from build123d import *

# Parameters (mm, degrees)
SKETCH2_R               = 95
SKETCH2_R_2             = 75
BOSS_EXTRUDE1_DEPTH     = 5
SKETCH3_R               = 87
SKETCH3_R_2             = 84
BOSS_EXTRUDE2_DEPTH     = 10
SKETCH4_R               = 78
SKETCH4_R_2             = 75
BOSS_EXTRUDE3_DEPTH     = 70
CUT_EXTRUDE3_DEPTH      = 161.23420359
CUT_EXTRUDE3_DEPTH_BACK = 161.23420359
SKETCH6_W               = 10
SKETCH6_H               = 12
CUT_EXTRUDE4_DEPTH      = 161.23420359
CUT_EXTRUDE4_DEPTH_BACK = 161.23420359
SKETCH7_W               = 10
SKETCH7_H               = 12


with BuildPart() as part:
    # Sketch2 → Boss-Extrude1 (new body)
    with BuildSketch(Plane.XY):
        Circle(SKETCH2_R)
        Circle(SKETCH2_R_2, mode=Mode.SUBTRACT)
    extrude(amount=BOSS_EXTRUDE1_DEPTH)

    # Sketch3 → Boss-Extrude2 (add)
    with BuildSketch(Plane.XY):
        Circle(SKETCH3_R)
        Circle(SKETCH3_R_2, mode=Mode.SUBTRACT)
    extrude(amount=BOSS_EXTRUDE2_DEPTH)

    # Sketch4 → Boss-Extrude3 (add)
    with BuildSketch(Plane.XY.offset(5)):
        Circle(SKETCH4_R)
        Circle(SKETCH4_R_2, mode=Mode.SUBTRACT)
    extrude(amount=BOSS_EXTRUDE3_DEPTH)

    # Sketch6 → Cut-Extrude3 (cut, two sides: drawn at the far end of the back side and taken through both)
    with BuildSketch(Plane(origin=(10, 0, 0), x_dir=(0, 0, -1), z_dir=(1, 0, 0)).offset(-CUT_EXTRUDE3_DEPTH_BACK)):
        with Locations((-40, 40)):
            Rectangle(SKETCH6_W, SKETCH6_H)
    extrude(amount=CUT_EXTRUDE3_DEPTH + CUT_EXTRUDE3_DEPTH_BACK, mode=Mode.SUBTRACT)

    # Sketch7 → Cut-Extrude4 (cut, two sides: drawn at the far end of the back side and taken through both)
    with BuildSketch(Plane(origin=(10, 0, 0), x_dir=(0, 0, -1), z_dir=(1, 0, 0)).offset(-CUT_EXTRUDE4_DEPTH_BACK)):
        with Locations((-40, -40)):
            Rectangle(SKETCH7_W, SKETCH7_H)
    extrude(amount=CUT_EXTRUDE4_DEPTH + CUT_EXTRUDE4_DEPTH_BACK, mode=Mode.SUBTRACT)


solid = part.part
The listing builds one solid part. Answer for the finished solid, in the listing's coordinates (mm). A direction names the side the tool comes from. Round coordinates to 2 decimals unless told otherwise and drop trailing zeros. Write each loop counter-clockwise with the first axis right and the second up, starting at its lowest first coordinate (ties: lowest second). Pieces come first, ordered by that corner, then holes. Notation, with made-up numbers: (-22.75, 57.25) - (-7.75, 57.25) arc R12 ccw to (-7.75, 64.25) - close; hole circle Ø8 at (26, -24.75). An arc over 180 degrees is marked (long way). Use a Markdown table: item, result. Add a question column.
1. A tool of negligible diameter and unlimited length cuts with its end or side. For faces 1 (the face through (-41, 64, 75)), 2 (the face through (-65, -40, 35)), 3 (the face through (24.5, -74.3, 5)), from which of +Z, -Z, +X, -X, +Y, -Y can it reach the whole face along a straight path? Write none if from no direction.
2. For a pull along X with two mould halves and no side action, classify faces 4 (the face through (-65, 40, 35)), 5 (the face through (80.12, 25.23, 7.46)), 6 (the face through (-20.59, -92.74, 2.46)), 7 (the face through (71.537, 22.528, 36.975)) as +X half, -X half, draft (parallel to the pull), parting line (faces both ways), or undercut.
3. The part is cut by section D-D (y = -40.5). Write down the section's boundary in (x, z).
4. Consider line 1 (Y direction, x = 0, z = 8.05); line 2 (X direction, y = 61.5, z = 8.5); line 3 (Y direction, x = 0, z = 54). Determine where each line is inside the solid, lowest interval first.
5. Flat-ended cylindrical pins translate along their axes: P1, Ø3.5, axis at x = 68, z = 40, coming from the -Y side; P2, Ø3.5, axis at x = -68.5, z = 37.5, coming from the +Y side; P3, Ø5, axis at y = -36.5, z = 67, coming from the -X side. Find the tip coordinate at first contact, or state that the pin passes through.
6. The part is cut by section A-A (y = 0). Write down the section's boundary in (x, z).
7. The part is cut by section C-C (z = 38). Write down the section's boundary in (x, y).
Reported:
| question | item | result |
|---|---|---|
| 1 | face 1 | +Z, +X, -X, +Y, -Y |
| 1 | face 2 | +X, -X |
| 1 | face 3 | +Z |
| 2 | face 4 | draft |
| 2 | face 5 | undercut |
| 2 | face 6 | parting line |
| 2 | face 7 | undercut |
| 3 | outline | (-85.93, 0) - (-63.12, 0) - (-63.12, 35) - (-66.66, 35) - (-66.66, 5) - (-73.59, 5) - (-73.59, 10) - (-77, 10) - (-77, 5) - (-85.93, 5) - close; (-66.66, 45) - (-63.12, 45) - (-63.12, 75) - (-66.66, 75) - close; (63.12, 0) - (85.93, 0) - (85.93, 5) - (77, 5) - (77, 10) - (73.59, 10) - (73.59, 5) - (66.66, 5) - (66.66, 35) - (63.12, 35) - close; (63.12, 45) - (66.66, 45) - (66.66, 75) - (63.12, 75) - close |
| 4 | line 1 | -87 to -84, -78 to -75, 75 to 78, 84 to 87 |
| 4 | line 2 | -61.54 to -57.22, -47.98 to -42.93, 42.93 to 47.98, 57.22 to 61.54 |
| 4 | line 3 | -78 to -75, 75 to 78 |
| 5 | P1 | y = -34 |
| 5 | P2 | y = 34 |
| 5 | P3 | x = -70.2 |
| 6 | outline | (-95, 0) - (-75, 0) - (-75, 75) - (-78, 75) - (-78, 5) - (-84, 5) - (-84, 10) - (-87, 10) - (-87, 5) - (-95, 5) - close; (75, 0) - (95, 0) - (95, 5) - (87, 5) - (87, 10) - (84, 10) - (84, 5) - (78, 5) - (78, 75) - (75, 75) - close |
| 7 | outline | (-70.2, -34) - (-66.85, -34) arc R75 cw to (-66.85, 34) - (-70.2, 34) arc R78 ccw to start; (-62.99, -46) arc R78 ccw to (62.99, -46) - (59.24, -46) arc R75 cw to (-59.24, -46) - close; (-62.99, 46) - (-59.24, 46) arc R75 cw to (59.24, 46) - (62.99, 46) arc R78 ccw to start; (66.85, -34) - (70.2, -34) arc R78 ccw to (70.2, 34) - (66.85, 34) arc R75 cw to start |
